For this review, take the finished solid that the model builds, in its own axes (mm). A direction names the side the tool comes from. Coordinates: 2 decimals unless noted, no trailing zeros. Loops run counter-clockwise (first coordinate to the right, second up) from the corner with the lowest first, then second, coordinate; pieces in that order, holes last. Notation, with made-up numbers: (38, 44.5) - (70, 44.5) arc R14 cw to (70, 51.5) - close; hole circle Ø5 at (87.25, 29). An arc over 180 degrees is marked (long way). Answer as a JSON object with one key per item and string values. Group by question number.
Item 1: Clearance check with flat-ended pins moving along their axes: pin 1 (5 mm diameter, centred on y = 20, z = 14.5, fed in from -X); pin 2 (10 mm diameter, centred on x = 205.5, z = 12, fed in from -Y); pin 3 (1.5 mm diameter, centred on x = 255, z = 17.5, fed in from -Y) (3 decimals). State where each tip first meets the part, or that it passes through.
Item 2: We need section A-A (z = 12.5). Give the boundary of the cut face in (x, y) (3 decimals), then the cut area to 3 significant figures.
Item 3: Tool access review of faces 1 (the cylindrical face through (154.5, -6.35, 15.1)), 2 (the cylindrical face through (150.228, -9.093, 11.27)), 3 (the flat face through (-2.54, 13, 11)), 4 (the cylindrical face through (154.572, 34.493, 11.27)): name each direction out of +Z, -Z, +X, -X, +Y, -Y from which nothing blocks a thin tool from reaching the whole face with its end or side.
Item 4: To check wall thickness, follow line 1 (X direction, y = 16.5, z = 17.5); line 2 (X direction, y = 5.5, z = 1.25); line 3 (Y direction, x = 41.5, z = 2.75). State the ranges of each line that lie inside material, in increasing order.
from build123d import *

# Parameters (mm, degrees)
F1_DEPTH = 2.54
F2_DEPTH = 27.94
F4_DEPTH = 2.54
F5_R     = 2.53999


# Not quite as in the source:
# - a fillet or chamfer is up to 0.001 mm smaller than in the source, because OpenCascade refuses the exact size


with BuildPart() as f1:
    # F0 (on Top) → F1 (new body)
    with BuildSketch(Plane.XY):
        with BuildLine():
            Line((0, 25.4), (0, 0))
            ThreePointArc((0, 0), (152.4, -6.35), (304.8, 0))
            Line((304.8, 0), (304.8, 25.4))
            ThreePointArc((304.8, 25.4), (152.4, 31.75), (0, 25.4))
        make_face()
    extrude(amount=F1_DEPTH)

    # F0 (on Top) → F2 (join)
    with BuildSketch(Plane.XY):
        with BuildLine():
            Line((-2.54, 27.94), (-2.54, -2.54))
            ThreePointArc((-2.54, -2.54), (152.4, -9.0943273232), (307.34, -2.54))
            Line((307.34, -2.54), (307.34, 27.94))
            ThreePointArc((307.34, 27.94), (152.4, 34.4943273232), (-2.54, 27.94))
        make_face()
        with BuildLine():
            ThreePointArc((304.8, 0), (152.4, -6.35), (0, 0))
            Line((0, 0), (0, 25.4))
            ThreePointArc((0, 25.4), (152.4, 31.75), (304.8, 25.4))
            Line((304.8, 25.4), (304.8, 0))
        make_face(mode=Mode.SUBTRACT)
    extrude(amount=F2_DEPTH)

    # F3 (on face) → F4 (join)
    with BuildSketch(Plane.XY.offset(27.94)):
        with BuildLine():
            ThreePointArc((309.88, 30.48), (152.4, 37.2416066482), (-5.08, 30.48))
            Line((-5.08, 30.48), (-5.08, -5.08))
            ThreePointArc((-5.08, -5.08), (152.4, -11.8416066482), (309.88, -5.08))
            Line((309.88, -5.08), (309.88, 30.48))
        make_face()
        with BuildLine():
            ThreePointArc((-2.54, 27.94), (152.4, 34.4943273232), (307.34, 27.94))
            Line((307.34, 27.94), (307.34, -2.54))
            ThreePointArc((307.34, -2.54), (152.4, -9.0943273232), (-2.54, -2.54))
            Line((-2.54, -2.54), (-2.54, 27.94))
        make_face(mode=Mode.SUBTRACT)
    extrude(amount=-F4_DEPTH)

    # F5 (radius 2.54 in the source; OpenCascade refuses exactly that, so slightly less here)
    f5_edges = [f1.edges().sort_by_distance(p)[0] for p in [
        (152.4, -9.094327, 25.4),
        (307.34, 12.7, 25.4),
        (152.4, 34.494327, 25.4),
        (-2.54, 12.7, 25.4),
        (0, 25.4, 15.24),
        (152.4, 31.75, 2.54),
        (0, 12.7, 2.54),
        (0, 0, 15.24),
        (304.8, 12.7, 2.54),
        (152.4, -6.35, 2.54),
        (304.8, 25.4, 15.24),
        (304.8, 0, 15.24),
        (152.4, 31.75, 27.94),
        (0, 12.7, 27.94),
        (304.8, 12.7, 27.94),
        (152.4, -6.35, 27.94),
    ]]
    fillet(f5_edges, radius=F5_R)


solid = f1.part
Check sheet entries:
{
 "1": {"pin 1": "stops at x = -2.54", "pin 2": "stops at y = -8.46", "pin 3": "stops at y = -6.265"},
 "2": {"outline": "(-2.54, -2.54) arc R1834.617 ccw to (307.34, -2.54) - (307.34, 27.94) arc R1834.617 ccw to (-2.54, 27.94) - close; hole (0, 2.338) arc R2.54 ccw to (2.332, -0.193) arc R1831.975 ccw to (302.468, -0.193) arc R2.54 ccw to (304.8, 2.338) - (304.8, 23.062) arc R2.54 ccw to (302.468, 25.593) arc R1831.975 ccw to (2.332, 25.593) arc R2.54 ccw to (0, 23.062) - close", "area": "1,840 mm2"},
 "3": {"face 1": "+Z", "face 2": "-Z, -Y", "face 3": "-Z, -X, +Y, -Y", "face 4": "-Z, +Y"},
 "4": {"line 1": "x = -2.54 to 0, 304.8 to 307.34", "line 2": "x = -2.54 to 307.34", "line 3": "y = -5.74 to -1.46, 26.86 to 31.14"}
}
